Input: part model. Units: mm. Frame: model coordinates. Face numbers are marked on the shaded views. A direction names the side the tool comes from. Give positions to 0.01 mm unless a question says otherwise; leave off trailing zeros. Write each loop counter-clockwise with the first axis right and the second up, starting at its lowest first coordinate (ties: lowest second). Pieces come first, ordered by that corner, then holes. Notation, with made-up numbers: (26.25, 54) - (52.25, 54) arc R36 cw to (52.25, 89) - close; hole circle Ø10 at (39.5, 71). An arc over 180 degrees is marked (long way). Use a Markdown table: item, result. Add a question column.
1. Mould query, pull axis X, two halves, no side actions, for the marked faces 3, 4, 5 and 6. Classes: released by +X, released by -X, zero draft, split by the parting line, or undercut.
2. Section query A-A, the plane z = 3.5. Return loops of the section in (x, y), plus the area to 3 significant figures.
3. Pin query (flat end, axial travel): pin 1 (5 mm diameter, centred on y = -8.5, z = 11.5, fed in from +X); pin 2 (1.6 mm diameter, centred on x = -51, y = -46, fed in from -Z); pin 3 (23.5 mm diameter, centred on x = -17.47, y = -21.32, fed in from -Z); pin 4 (2 mm diameter, centred on x = 16, y = -28.5, fed in from -Z). Return the tip coordinate at first contact, or that it passes through.
4. Material intervals for probe 1 along X at (y, z) = (-45.5, -4); probe 2 along Z at (x, y) = (3.5, -39); probe 3 along Z at (x, y) = (-40, -60), sorted ascending.
5. Set-up query: the marked faces 1 and 2. Return all of +Z, -Z, +X, -X, +Y, -Y with unobstructed straight access to the full face (end or side cutting, diameter ignored); none if empty.
6. Section query D-D, the plane y = -19.5. Return loops of the section in (x, z), plus the area to 3 significant figures.
7. Section query B-B, the plane y = -56.5. Return loops of the section in (x, z), plus the area to 3 significant figures.
8. Section query C-C, the plane y = -32.5. Return loops of the section in (x, z), plus the area to 3 significant figures.
```python
from build123d import *

# Parameters (mm, degrees)
F0_W     = 5.8722943068
F0_H     = 45.8038914949
F0_W_2   = 5.8722924441
F0_H_2   = 46.0975058377
F1_DEPTH = 76.2
F3_D     = 20.32


with BuildPart() as f1:
    # F0 (on Front) → F1 (new body)
    with BuildSketch(Plane.XZ):
        Polygon((-37.7294868231, 30.5359270424), (-53.8782961667, 30.5359270424), (-53.8782961667, 25.2508632839), (-48.5932305455, 25.2508632839), (-42.7209362388, 25.2508632839), (-37.7294868231, 25.2508632839), align=None)
        with Locations((-45.6570833921, 2.3489175364)):
            Rectangle(F0_W, F0_H)
        Polygon((-42.7209362388, -20.553028211), (-48.5932305455, -20.553028211), (-48.5932305455, -28.1870104373), (13.9466961846, -28.1870104373), (13.9466961846, -20.553028211), (8.0744037405, -20.553028211), align=None)
        with Locations((11.0105499625, 2.4957247078)):
            Rectangle(F0_W_2, F0_H_2)
        Polygon((3.3765700646, 25.5444776267), (8.0744037405, 25.5444776267), (13.9466961846, 25.5444776267), (18.350917846, 25.5444776267), (18.350917846, 30.5359270424), (3.3765700646, 30.5359270424), align=None)
    extrude(amount=F1_DEPTH)

    # F3 (through all)
    with Locations(Plane.XY.offset(-20.553028211)):
        with Locations((-17.4700734206, -21.3164253719), (-17.4700734206, -61.3654702902)):
            Hole(F3_D / 2)


solid = f1.part
```
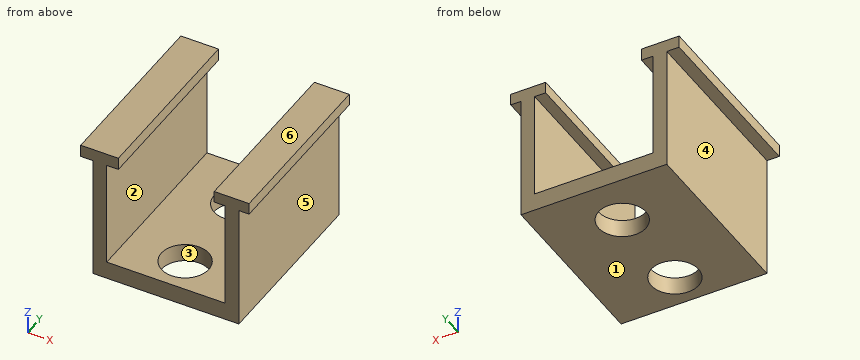
Result sheet:
| question | item | result |
|---|---|---|
| 1 | face 3 | undercut |
| 1 | face 4 | released by -X |
| 1 | face 5 | released by +X |
| 1 | face 6 | zero draft |
| 2 | outline | (-48.59, -76.2) - (-42.72, -76.2) - (-42.72, 0) - (-48.59, 0) - close; (8.07, -76.2) - (13.95, -76.2) - (13.95, 0) - (8.07, 0) - close |
| 2 | area | 895 mm² |
| 3 | pin 1 | stops at x = 13.95 |
| 3 | pin 2 | stops at z = 25.25 |
| 3 | pin 3 | stops at z = -28.19 |
| 3 | pin 4 | stops at z = 25.54 |
| 4 | probe 1 | x = -48.59 to -42.72, 8.07 to 13.95 |
| 4 | probe 2 | z = -28.19 to -20.55, 25.54 to 30.54 |
| 4 | probe 3 | z = -28.19 to -20.55, 25.25 to 30.54 |
| 5 | face 1 | -Z, +X, -X, +Y, -Y |
| 5 | face 2 | +Y, -Y |
| 6 | outline | (-53.88, 25.25) - (-48.59, 25.25) - (-48.59, -28.19) - (-27.47, -28.19) - (-27.47, -20.55) - (-42.72, -20.55) - (-42.72, 25.25) - (-37.73, 25.25) - (-37.73, 30.54) - (-53.88, 30.54) - close; (-7.47, -28.19) - (13.95, -28.19) - (13.95, 25.54) - (18.35, 25.54) - (18.35, 30.54) - (3.38, 30.54) - (3.38, 25.54) - (8.07, 25.54) - (8.07, -20.55) - (-7.47, -20.55) - close |
| 6 | area | 1,020 mm² |
| 7 | outline | (-53.88, 25.25) - (-48.59, 25.25) - (-48.59, -28.19) - (-26.39, -28.19) - (-26.39, -20.55) - (-42.72, -20.55) - (-42.72, 25.25) - (-37.73, 25.25) - (-37.73, 30.54) - (-53.88, 30.54) - close; (-8.55, -28.19) - (13.95, -28.19) - (13.95, 25.54) - (18.35, 25.54) - (18.35, 30.54) - (3.38, 30.54) - (3.38, 25.54) - (8.07, 25.54) - (8.07, -20.55) - (-8.55, -20.55) - close |
| 7 | area | 1,040 mm² |
| 8 | outline | (-53.88, 25.25) - (-48.59, 25.25) - (-48.59, -28.19) - (13.95, -28.19) - (13.95, 25.54) - (18.35, 25.54) - (18.35, 30.54) - (3.38, 30.54) - (3.38, 25.54) - (8.07, 25.54) - (8.07, -20.55) - (-42.72, -20.55) - (-42.72, 25.25) - (-37.73, 25.25) - (-37.73, 30.54) - (-53.88, 30.54) - close |
| 8 | area | 1,180 mm² |
